```python
from build123d import *

# Parameters (mm, degrees)
F1_DEPTH = 30
F2_DEPTH = 10
F3_DEPTH = 20
F5_DEPTH = 10.001


with BuildPart() as f1:
    # F0 (on Front) → F1 (new body)
    with BuildSketch(Plane.XZ):
        Polygon((0, 28), (0, 5), (10, 5), (10, 17), (10, 28), align=None)
        Polygon((0, 5), (0, 0), (50, 0), (50, 5), (21, 5), (21, 17), (10, 17), (10, 5), align=None)
        Polygon((21, 5), (50, 5), (50, 11), (39.764706, 17), (21, 17), align=None)
        Polygon((21, 28), (10, 28), (10, 17), (21, 17), (39.764706, 17), align=None)
    extrude(amount=-F1_DEPTH)

    # F0 (on Front) → F2 (cut)
    with BuildSketch(Plane.XZ):
        Polygon((0, 5), (0, 0), (50, 0), (50, 5), (21, 5), (21, 17), (10, 17), (10, 5), align=None)
    extrude(amount=-F2_DEPTH, mode=Mode.SUBTRACT)

    # F0 (on Front) → F3 (cut)
    with BuildSketch(Plane.XZ):
        Polygon((21, 28), (10, 28), (10, 17), (21, 17), (39.764706, 17), align=None)
    extrude(amount=-F3_DEPTH, mode=Mode.SUBTRACT)

    # F4 (on face) → F5 (cut, through all)
    with BuildSketch(Plane.YZ.offset(10)):
        Polygon((0, 17), (10, 28), (0, 28), align=None)
    extrude(amount=-F5_DEPTH, mode=Mode.SUBTRACT)


solid = f1.part
```
Geometry check sheet. Reference: the model listing, model coordinates, mm. A direction names the side the tool comes from. Give positions to 0.01 mm unless a question says otherwise; leave off trailing zeros. Write each loop counter-clockwise with the first axis right and the second up, starting at its lowest first coordinate (ties: lowest second). Pieces come first, ordered by that corner, then holes. Notation, with made-up numbers: (21.25, 84.25) -> (48.25, 84.25) arc R22 cw to (48.25, 123.25) -> close; hole circle Ø7 at (70.25, -8.5). An arc over 180 degrees is marked (long way). One line per question, with ' | ' between items.
Item 1: Sectioned sample at C-C, the plane y = 18.25. Record the boundary of the cut face in (x, z), plus the area to 3 significant figures.
Determined:
outline: (0, 0) -> (50, 0) -> (50, 11) -> (39.76, 17) -> (10, 17) -> (10, 28) -> (0, 28) -> close | area: 929 mm^2
Item 2: Access from +Z, -Z, +X, -X, +Y, -Y to the whole of each face (thin tool, end or side, straight path). Record for faces 1 (the flat face through (5, 5, 5)), 2 (the flat face through (21, 5, 11)), 3 (the flat face through (28, 10, 17)), 4 (the flat face through (10, 8, 17)).
Determined:
face 1: -Z, +X, -X, -Y | face 2: +Z, -Z, -Y | face 3: +Z, +X, -Y | face 4: +Z, -Y
Item 3: Sectioned sample at A-A, the plane y = 2.5. Record the boundary of the cut face in (x, z).
Determined:
outline: (0, 5) -> (10, 5) -> (10, 19.75) -> (0, 19.75) -> close; (21, 5) -> (50, 5) -> (50, 11) -> (39.76, 17) -> (21, 17) -> close
Item 4: Draft check along X on faces 5 (the flat face through (24.7, 10, 4.8)), 6 (the flat face through (36, 5, 5)), 7 (the flat face through (0, 18, 14)). Enter one of: released by +X, released by -X, zero draft, split by the parting line, or undercut.
Determined:
face 5: undercut | face 6: zero draft | face 7: released by -X
Item 5: Sectioned sample at D-D, the plane z = 9.5. Record the boundary of the cut face in (x, y).
Determined:
outline: (0, 0) -> (10, 0) -> (10, 10) -> (21, 10) -> (21, 0) -> (50, 0) -> (50, 30) -> (0, 30) -> close
Item 6: Sectioned sample at B-B, the plane x = 6. Record the boundary of the cut face in (y, z), plus the area to 3 significant figures.
Determined:
outline: (0, 5) -> (10, 5) -> (10, 0) -> (30, 0) -> (30, 28) -> (10, 28) -> (0, 17) -> close | area: 735 mm^2
Item 7: Depth check by flat-ended pin: pin 1 (11 mm diameter, centred on x = 30, y = 3, fed in from -Z); pin 2 (6 mm diameter, centred on x = 28, y = 7.5, fed in from +Z); pin 3 (5.5 mm diameter, centred on x = 20, z = 23.5, fed in from -Y). Enter the tip coordinate at first touch or a pass-through.
Determined:
pin 1: z = 5 | pin 2: z = 17 | pin 3: y = 20
Item 8: Scan lines: line 1 along X through (y, z) = (3, 10.5); line 2 along X through (y, z) = (16.25, 22.25); line 3 along Z through (x, y) = (14.5, 15). Record each from-to range of solid material in increasing order.
Determined:
line 1: 0 to 10, 21 to 50 | line 2: 0 to 10 | line 3: 0 to 17
